```python
from build123d import *

# Parameters (mm, degrees)
SKETCH3_R          = 1.6
CUT_EXTRUDE1_DEPTH = 18
CIRPATTERN1_COUNT  = 4


with BuildPart() as part:
    # Sketch2 → Revolve1 (revolve)
    with BuildSketch(Plane.XY):
        Polygon((15, 50), (-15, 50), (-15, 35), (-2, 35), (-2, 25), (2, 25), (2, 35), (15, 35), align=None)
    revolve(axis=Axis((0, 0, 0), (1, 0, 0)))

    # Sketch3 → Cut-Extrude1 (cut, through all)
    with BuildSketch(Plane(origin=(2, 0, 0), x_dir=(0, 0, -1), z_dir=(1, 0, 0))):
        with Locations((0, 30)):
            Circle(SKETCH3_R)
    cut_extrude1 = extrude(amount=-CUT_EXTRUDE1_DEPTH, mode=Mode.SUBTRACT)

    # CirPattern1: Cut-Extrude1 ×4 about axis
    cirpattern1_axis = Axis((0, 0, 0), (1, 0, 0))
    for i in range(1, CIRPATTERN1_COUNT):
        add(cut_extrude1.rotate(cirpattern1_axis, i * 360 / CIRPATTERN1_COUNT), mode=Mode.SUBTRACT)


solid = part.part
```
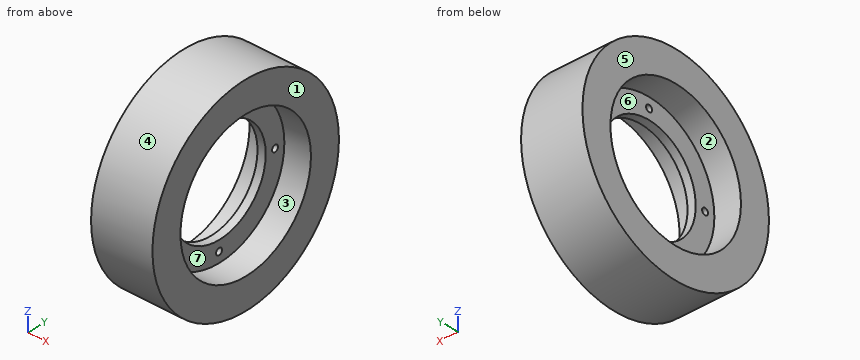
Verification items for the finished model (mm, model axes). Face numbers are marked on the shaded views. A direction names the side the tool comes from. Give positions to 0.01 mm unless a question says otherwise; leave off trailing zeros. Order: outer loops, then holes, each group sorted by start corner. A loop starts at its lowest first (then second) coordinate and runs counter-clockwise, first axis right, second up. Notation, with made-up numbers: M 16,-10 L 69,-10 A25 cw 69,26 Z; hole C 78,46.5 d8. An arc over 180 degrees is marked long. Return JSON: item names as keys, results as strings. Group by question number.
1) Go/stop test with flat-tipped pins: pin 1 Ø2 at (y, z) = (-32, 8.5) entering from -X; pin 2 Ø3.5 at (y, z) = (-30, 0) entering from +X; pin 3 Ø1.5 at (x, z) = (11.5, -24) entering from -Y. Record where each tip stops, or that it passes through.
2) Scan lines: line 1 (Z direction, x = -0.75, y = 0); line 2 (X direction, y = -5, z = 28); line 3 (Y direction, x = -4, z = 8). Record each from-to range of solid material in increasing order.
3) Mould release check, pull along Z, two halves, no side actions. Record for the marked faces 4, 5, 6 and 7: pulls with the +Z half, pulls with the -Z half, needs draft (parallel to the pull), parting line crosses it, or undercut.
4) Section check C-C on x = 0.25. Record the cut outline in (y, z), and give its area (3 significant figures).
5) Section check D-D on y = 22.5. Record the cut outline in (x, z).
6) Section check A-A on z = 0. Record the cut outline in (x, y), and give its area (3 significant figures).
7) Access from +Z, -Z, +X, -X, +Y, -Y to the whole of each face (thin tool, end or side, straight path). Record for the marked faces 1, 2 and 3.
Answer block:
{
 "1": {"pin 1": "stops at x = -2", "pin 2": "stops at x = 2", "pin 3": "stops at y = -44.27"},
 "2": {"line 1": "z = -50 to -31.6, -28.4 to -25, 25 to 28.4, 31.6 to 50", "line 2": "x = -2 to 2", "line 3": "y = -49.36 to -34.07, 34.07 to 49.36"},
 "3": {"face 4": "parting line crosses it", "face 5": "needs draft", "face 6": "undercut", "face 7": "undercut"},
 "4": {"outline": "C 0,0 d100; hole C -30,0 d3.2; hole C 0,0 d50; hole C 0,-30 d3.2; hole C 0,30 d3.2; hole C 30,0 d3.2", "area": "5,860 mm^2"},
 "5": {"outline": "M -15,-44.65 L 15,-44.65 L 15,-26.81 L 2,-26.81 L 2,-10.9 L -2,-10.9 L -2,-26.81 L -15,-26.81 Z; M -15,26.81 L -2,26.81 L -2,10.9 L 2,10.9 L 2,26.81 L 15,26.81 L 15,44.65 L -15,44.65 Z"},
 "6": {"outline": "M -15,-50 L 15,-50 L 15,-35 L 2,-35 L 2,-31.6 L -2,-31.6 L -2,-35 L -15,-35 Z; M -15,35 L -2,35 L -2,31.6 L 2,31.6 L 2,35 L 15,35 L 15,50 L -15,50 Z; M -2,-28.4 L 2,-28.4 L 2,-25 L -2,-25 Z; M -2,25 L 2,25 L 2,28.4 L -2,28.4 Z", "area": "954 mm^2"},
 "7": {"face 1": "+Z, -Z, +X, +Y, -Y", "face 2": "-X", "face 3": "+X"}
}
